from build123d import *

# Parameters (mm, degrees)
SKETCH1_W           = 41.91
SKETCH1_H           = 50.8
BOSS_EXTRUDE1_DEPTH = 41.91
SKETCH2_R           = 17.78
BOSS_EXTRUDE2_DEPTH = 43.18
BOSS_EXTRUDE4_DEPTH = 43.18


with BuildPart() as part:
    # Sketch1 → Boss-Extrude1 (new body)
    with BuildSketch(Plane(origin=(0, 0, 0), x_dir=(1, 0, 0), z_dir=(0, 1, 0))):
        with Locations((-20.955, 25.4)):
            Rectangle(SKETCH1_W, SKETCH1_H)
    extrude(amount=BOSS_EXTRUDE1_DEPTH)

    # Sketch2 → Boss-Extrude2 (add)
    with BuildSketch(Plane(origin=(0, 0, -50.8), x_dir=(-1, 0, 0), z_dir=(0, 0, -1))):
        with Locations((20.955, 20.955)):
            Circle(SKETCH2_R)
    extrude(amount=BOSS_EXTRUDE2_DEPTH)

    # Sketch3 → Boss-Extrude4 (add)
    with BuildSketch(Plane.XY):
        Polygon((-13.622651581, 20.955), (-17.288825791, 27.305), (-24.621174209, 27.305), (-28.287348419, 20.955), (-24.621174209, 14.605), (-17.288825791, 14.605), align=None)
    extrude(amount=BOSS_EXTRUDE4_DEPTH)


solid = part.part
The listing builds one solid part. Answer for the finished solid, in the listing's coordinates (mm). A direction names the side the tool comes from. Round coordinates to 2 decimals unless told otherwise and drop trailing zeros. Order: outer loops, then holes, each group sorted by start corner. A loop starts at its lowest first (then second) coordinate and runs counter-clockwise, first axis right, second up. Notation, with made-up numbers: (83.5, 78.5) - (117.5, 78.5) arc R16 cw to (117.5, 105.5) - close; hole circle Ø6 at (51.25, 16.25). An arc over 180 degrees is marked (long way). Write item = value, one per line. Start each with the question number.
1) Given pin 1 (3.5 mm diameter, centred on x = -22.5, z = 16, fed in from +Y) (3 decimals); pin 2 (8 mm diameter, centred on x = -36.5, y = 34.5, fed in from +Z); pin 3 (3.5 mm diameter, centred on x = -22.5, z = 17.5, fed in from -Y) (3 decimals), each flat-ended and moving along its own axis, determine where each tip first touches the part or whether it passes through.
2) For faces 1 (the flat face through (-21, 27.305, 21)), 2 (the flat face through (-26, 16, 0)), 3 (the flat face through (-15.43, 24.086, 21.288)), 4 (the flat face through (-15.5, 17.7, 21.3)), determine the directions among +Z, -Z, +X, -X, +Y, -Y from which every point of the face is accessible in a straight line to the end or side of a thin tool.
3) Section D-D, the plane y = 35.5 is taken. Write down the section's boundary in (x, z), plus the area to 3 significant figures.
4) Section C-C, the plane z = -72.5 is taken. Write down the section's boundary in (x, y) (3 decimals), plus the area to 3 significant figures.
5) Section B-B, the plane x = -20 is taken. Write down the section's boundary in (y, z) (3 decimals), plus the area to 3 significant figures.
6) Section A-A, the plane y = 24 is taken. Write down the section's boundary in (x, z), plus the area to 3 significant figures.
7) Straight lines are drawn through the part: L1, parallel to Z at x = -21, y = 35; L2, parallel to Z at x = -31, y = 5.5; L3, parallel to Y at x = -20.5, z = 13 (3 decimals). For each, find the intervals that lie inside material, in ascending order.
Results list:
q1.pin_1 = 27.305
q1.pin_2 = 0
q1.pin_3 = 14.605
q2.face_1 = +Z, +X, -X, +Y
q2.face_2 = +Z
q2.face_3 = +Z, +X, +Y
q2.face_4 = +Z, +X, -Y
q3.outline = (-41.91, -50.8) - (-31.18, -50.8) - (-31.18, -93.98) - (-10.73, -93.98) - (-10.73, -50.8) - (0, -50.8) - (0, 0) - (-41.91, 0) - close
q3.area = 3,010 mm^2
q4.outline = circle Ø35.56 at (-20.955, 20.955)
q4.area = 993 mm^2
q5.outline = (0, -50.8) - (3.201, -50.8) - (3.201, -93.98) - (38.709, -93.98) - (38.709, -50.8) - (41.91, -50.8) - (41.91, 0) - (27.305, 0) - (27.305, 43.18) - (14.605, 43.18) - (14.605, 0) - (0, 0) - close
q5.area = 4,210 mm^2
q6.outline = (-41.91, -50.8) - (-38.47, -50.8) - (-38.47, -93.98) - (-3.44, -93.98) - (-3.44, -50.8) - (0, -50.8) - (0, 0) - (-15.38, 0) - (-15.38, 43.18) - (-26.53, 43.18) - (-26.53, 0) - (-41.91, 0) - close
q6.area = 4,120 mm^2
q7.L1 = -93.98 to 0
q7.L2 = -50.8 to 0
q7.L3 = 14.605 to 27.305
